For this review, use the dimensioned drawing (mm, ordinates from the lowest corner) and the shaded views. Coordinates: 2 decimals unless noted, no trailing zeros. Loops run counter-clockwise (first coordinate to the right, second up) from the corner with the lowest first, then second, coordinate; pieces in that order, holes last. Notation, with made-up numbers: (68.5, -5) - (94.5, -5) arc R25 cw to (94.5, 34) - close; hole circle Ø6 at (-25, 85). An arc over 180 degrees is marked (long way). Answer in a Markdown table with one row per item. Add a question column.
(1) We need section D-D on y = 6.5. Write out the cut boundary in (x, z), plus the area to 3 significant figures.
(2) We need section B-B on z = 37. Write out the cut boundary in (x, y).
(3) For P1, Ø6, axis at x = 5.5, y = 13, coming from the +Z side; P2, Ø3, axis at y = 5, z = 57, coming from the +X side; P3, Ø3, axis at x = 15, z = 57, coming from the +Y side; P4, Ø4, axis at x = 28, z = 13.5, coming from the -Y side, all flat-tipped, find the tip position at first contact; note any pin that passes through.
(4) Mouldability with a two-part tool opening along Z and no side actions: class the marked faces 1, 2 and 3 as +Z half, -Z half, draft (parallel to the pull), parting line (faces both ways), or undercut.
(5) We need section A-A on y = 13. Write out the cut boundary in (x, z).
(6) For line 1 along Z through (x, y) = (17, 11.75); line 2 along X through (y, z) = (7.25, 42.5); line 3 along Y through (x, z) = (18.5, 24), list the stretches that pass through material, from the lowest coordinate up.
(7) We need section C-C on x = 29.21. Write out the cut boundary in (y, z).
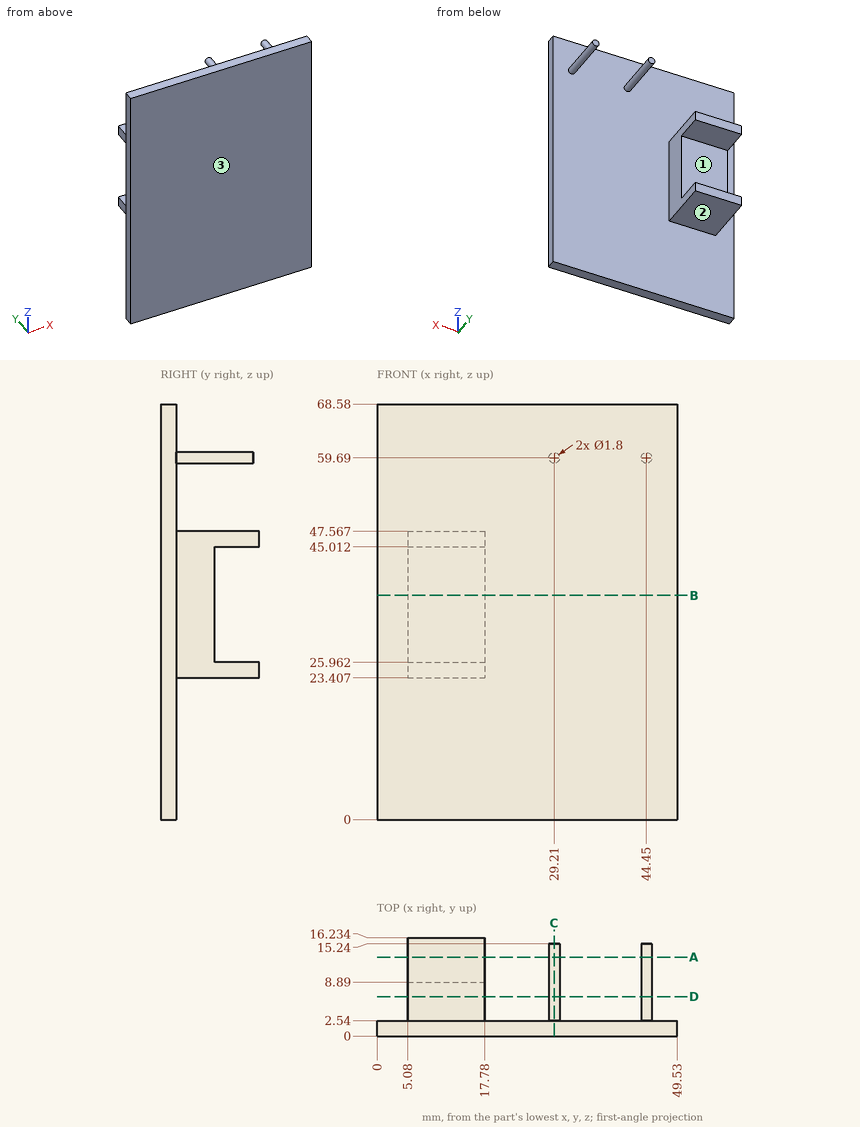
Outcome:
| question | item | result |
|---|---|---|
| 1 | outline | (5.08, 23.41) - (17.78, 23.41) - (17.78, 47.57) - (5.08, 47.57) - close; circle Ø1.8 at (29.21, 59.69); circle Ø1.8 at (44.45, 59.69) |
| 1 | area | 312 mm² |
| 2 | outline | (0, 0) - (49.53, 0) - (49.53, 2.54) - (17.78, 2.54) - (17.78, 8.89) - (5.08, 8.89) - (5.08, 2.54) - (0, 2.54) - close |
| 3 | P1 | z = 47.57 |
| 3 | P2 | through |
| 3 | P3 | y = 2.54 |
| 3 | P4 | y = 0 |
| 4 | face 1 | undercut |
| 4 | face 2 | -Z half |
| 4 | face 3 | draft |
| 5 | outline | (5.08, 23.41) - (17.78, 23.41) - (17.78, 25.96) - (5.08, 25.96) - close; (5.08, 45.01) - (17.78, 45.01) - (17.78, 47.57) - (5.08, 47.57) - close; circle Ø1.8 at (29.21, 59.69); circle Ø1.8 at (44.45, 59.69) |
| 6 | line 1 | 23.41 to 25.96, 45.01 to 47.57 |
| 6 | line 2 | 5.08 to 17.78 |
| 6 | line 3 | 0 to 2.54 |
| 7 | outline | (0, 0) - (2.54, 0) - (2.54, 58.79) - (15.24, 58.79) - (15.24, 60.59) - (2.54, 60.59) - (2.54, 68.58) - (0, 68.58) - close |
